Solid Edge part; units mm, degrees
sketch "Sketch1" plane through (0, 0, 0) normal (0, 0, 1) x (1, 0, 0)
  line L0 (1077.6266, -622.6959) -> (483.7062, -279.7959)
  line L1 (0.4572, -1244.6) -> (0.4572, -558.7998)
  line L2 (0.4572, -1244.6) -> (0.4572, -1930.3999)
  line L3 (1077.6266, -622.6959) -> (1671.5468, -965.5959)
  arc A0 (483.7062, -279.7959) -> (0.4572, -558.7998) centre (0, 0) cw
  arc A1 (1671.5468, -965.5959) -> (0.4572, -1930.3999) centre (0, 0) cw
  circle A2 centre (622.3, -1077.8552) radius 571.5
extrude "Protrusion1" add sketch "Sketch1" along normal blind 12.7
chamfer "Chamfer_1" distance 3.175 angle 45 1 edges at (50.8, -1077.8552, 12.7)
chamfer "Chamfer_2" distance 6.35 angle 45 1 edges at (50.8, -1077.8552, 0)
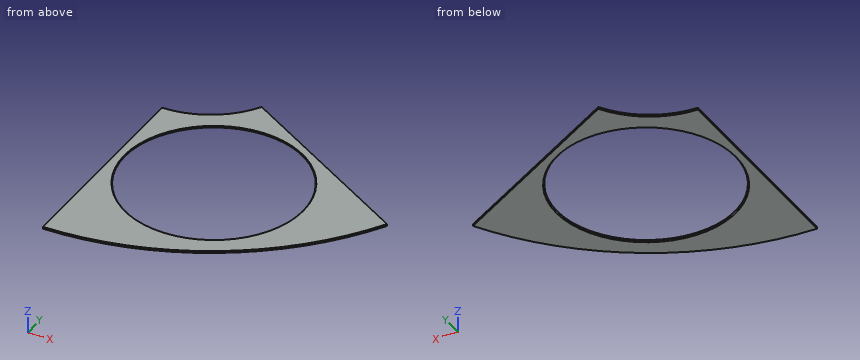
For this review, take the finished solid that the model builds, in its own axes (mm). Coordinates: 2 decimals unless noted, no trailing zeros. Write each loop counter-clockwise with the first axis right and the second up, starting at its lowest first coordinate (ties: lowest second). Pieces come first, ordered by that corner, then holes.
(1) Add section A-A on x = 622.3. Give the boundary of the cut face in (y, z) (3 decimals), then the cut area to 3 significant figures.
(2) Add section C-C on x = 1446. Give the boundary of the cut face in (y, z).
(3) For pin 1 Ø5 at (x, z) = (1405, 9) entering from +Y; pin 2 Ø4 at (x, z) = (473, 10.5) entering from +Y; pin 3 Ø2 at (y, z) = (-1248, 2) entering from +X, all flat-tipped, find the tip position at first contact; note any pin that passes through.
(4) Wall thickness on probe 1 along X at (y, z) = (-1124, 8.75); probe 2 along X at (y, z) = (-609, 10.5); probe 3 along Y at (x, z) = (904, 7.75) (3 decimals): over which ranges is each line inside the solid? List them lowest first.
(5) Add section B-B on z = 3.5. Give the boundary of the cut face in (x, y), then the cut area to 3 significant figures.
Answer sheet:
1. outline: (-1827.344, 0) - (-1655.705, 0) - (-1649.355, 6.35) - (-1649.355, 9.525) - (-1652.53, 12.7) - (-1827.344, 12.7) - close; (-506.355, 6.35) - (-500.005, 0) - (-359.813, 0) - (-359.813, 12.7) - (-503.18, 12.7) - (-506.355, 9.525) - close
1. area: 4,070 mm2
2. outline: (-1278.88, 0) - (-835.38, 0) - (-835.38, 12.7) - (-1278.88, 12.7) - close
3. pin 1: stops at y = -810.26
3. pin 2: stops at y = -294.33
3. pin 3: stops at x = 1473.58
4. probe 1: x = 0.46 to 52.67, 1191.93 to 1569.42
4. probe 2: x = 0.46 to 293.81, 950.79 to 1053.9
4. probe 3: y = -1705.646 to -1575.105, -580.605 to -522.453
5. outline: (0.46, -1930.4) arc R1930.4 ccw to (1671.55, -965.6) - (1077.63, -622.7) - (483.71, -279.8) arc R558.8 cw to (0.46, -558.8) - close; hole circle Ø1148.7 at (622.3, -1077.86)
5. area: 750,000 mm2
